Could you check a few things on this model? Use its own coordinates, in mm. A direction names the side the tool comes from. Give positions to 0.01 mm unless a question says otherwise; leave off trailing zeros. Loops run counter-clockwise (first coordinate to the right, second up) from the corner with the lowest first, then second, coordinate; pieces in that order, holes last. Notation, with made-up numbers: (-0.5, 24) - (36.5, 24) arc R34 cw to (36.5, 61) - close; hole circle Ø8 at (-14.5, 68.25). An arc over 180 degrees is marked (long way). Use CSV: the item, a comma, the result in double quotes.
from build123d import *
from OCP.BRepFilletAPI import BRepFilletAPI_MakeChamfer

# Parameters (mm, degrees)
SKIZZE1_R                            = 35
AUFSATZ_LINEAR_AUSTRAGEN1_DEPTH      = 10
SKIZZE1_3_OUTSIDE_W                  = 91.9
SKIZZE1_3_OUTSIDE_H                  = 91.9
SKIZZE1_3_OUTSIDE_R                  = 35
SKIZZE1_3_OUTSIDE_W_2                = 15.1
SKIZZE1_3_OUTSIDE_H_2                = 20.2
SCHNITT_LINEAR_AUSTRAGEN1_DEPTH      = 10
SCHNITT_LINEAR_AUSTRAGEN2_DEPTH      = 1
SCHNITT_LINEAR_AUSTRAGEN2_DEPTH_BACK = 8
SKIZZE2_R                            = 5.1
SKIZZE3_R                            = 32.5
SKIZZE3_R_2                          = 30.5
AUFSATZ_LINEAR_AUSTRAGEN2_DEPTH      = 1
SKIZZE4_R                            = 15.137010129
SKIZZE4_R_2                          = 12.637010129
AUFSATZ_LINEAR_AUSTRAGEN3_DEPTH      = 1
FASE1_SIZE                           = 1
FASE1_SIZE2                          = 5.67128182


with BuildPart() as part:
    # Skizze1 → Aufsatz-Linear austragen1 (new body)
    with BuildSketch(Plane.XY):
        Circle(SKIZZE1_R)
    extrude(amount=AUFSATZ_LINEAR_AUSTRAGEN1_DEPTH)

    # Skizze1_3 outside → Schnitt-Linear austragen1 (cut)
    # profile 1 of 2: a face of its own
    with BuildSketch(Plane.XY):
        Rectangle(SKIZZE1_3_OUTSIDE_W, SKIZZE1_3_OUTSIDE_H)
        Circle(SKIZZE1_3_OUTSIDE_R, mode=Mode.SUBTRACT)
    # profile 2 of 2: a face of its own
    with BuildSketch(Plane.XY):
        with Locations((0.045, 0)):
            Rectangle(SKIZZE1_3_OUTSIDE_W_2, SKIZZE1_3_OUTSIDE_H_2)
    extrude(amount=SCHNITT_LINEAR_AUSTRAGEN1_DEPTH, mode=Mode.SUBTRACT)

    # Skizze2 → Schnitt-Linear austragen2 (cut, two sides: drawn at the far end of the back side and taken through both)
    with BuildSketch(Plane(origin=(0, 0, 0), x_dir=(-1, 0, 0), z_dir=(0, 0, -1)).offset(-SCHNITT_LINEAR_AUSTRAGEN2_DEPTH_BACK)):
        with Locations(Location((0, 25, 0), (0, 0, 180))):
            Circle(SKIZZE2_R)
    extrude(amount=SCHNITT_LINEAR_AUSTRAGEN2_DEPTH + SCHNITT_LINEAR_AUSTRAGEN2_DEPTH_BACK, mode=Mode.SUBTRACT)

    # Skizze3 → Aufsatz-Linear austragen2 (add)
    with BuildSketch(Plane.XY.offset(10)):
        Circle(SKIZZE3_R)
        Circle(SKIZZE3_R_2, mode=Mode.SUBTRACT)
    extrude(amount=AUFSATZ_LINEAR_AUSTRAGEN2_DEPTH)

    # Skizze4 → Aufsatz-Linear austragen3 (add)
    with BuildSketch(Plane.XY.offset(10)):
        Circle(SKIZZE4_R)
        with Locations(Location((0, 0, 0), (0, 0, 53.057558872))):
            Circle(SKIZZE4_R_2, mode=Mode.SUBTRACT)
    extrude(amount=AUFSATZ_LINEAR_AUSTRAGEN3_DEPTH)

    # Fase1: one chamfer whose edges measure the first distance from different faces: ONE call of the kernel's chamfer builder (chamfer() names one face for all edges)
    fase1_edges_1 = [part.edges().sort_by_distance(p)[0] for p in [
        (-7.505, 0, 0),
    ]]
    fase1_side_1 = [part.faces().sort_by_distance(p)[0] for p in [
        (-7.505, 0, 5),
    ]]
    fase1_edges_2 = [part.edges().sort_by_distance(p)[0] for p in [
        (0.045, -10.1, 0),
    ]]
    fase1_side_2 = [part.faces().sort_by_distance(p)[0] for p in [
        (0.045, -10.1, 5),
    ]]
    fase1_edges_3 = [part.edges().sort_by_distance(p)[0] for p in [
        (7.595, 0, 0),
    ]]
    fase1_side_3 = [part.faces().sort_by_distance(p)[0] for p in [
        (7.595, 0, 5),
    ]]
    fase1_edges_4 = [part.edges().sort_by_distance(p)[0] for p in [
        (0.045, 10.1, 0),
    ]]
    fase1_side_4 = [part.faces().sort_by_distance(p)[0] for p in [
        (0.045, 10.1, 5),
    ]]
    fase1 = BRepFilletAPI_MakeChamfer(part.part.solid().wrapped)
    for e in fase1_edges_1:
        fase1.Add(FASE1_SIZE, FASE1_SIZE2, e.wrapped, fase1_side_1[0].wrapped)  # the first distance lies on this face
    for e in fase1_edges_2:
        fase1.Add(FASE1_SIZE, FASE1_SIZE2, e.wrapped, fase1_side_2[0].wrapped)  # the first distance lies on this face
    for e in fase1_edges_3:
        fase1.Add(FASE1_SIZE, FASE1_SIZE2, e.wrapped, fase1_side_3[0].wrapped)  # the first distance lies on this face
    for e in fase1_edges_4:
        fase1.Add(FASE1_SIZE, FASE1_SIZE2, e.wrapped, fase1_side_4[0].wrapped)  # the first distance lies on this face
    add(Compound.cast(fase1.Shape()), mode=Mode.REPLACE)


solid = part.part
1) Suppose I cut it at B-B (y = 0). Please give me the cut outline in (x, z) (3 decimals).
Answer below:
outline,"(-35, 0) - (-13.176, 0) - (-7.505, 1) - (-7.505, 10) - (-12.637, 10) - (-12.637, 11) - (-15.137, 11) - (-15.137, 10) - (-30.5, 10) - (-30.5, 11) - (-32.5, 11) - (-32.5, 10) - (-35, 10) - close; (7.595, 1) - (13.266, 0) - (35, 0) - (35, 10) - (32.5, 10) - (32.5, 11) - (30.5, 11) - (30.5, 10) - (15.137, 10) - (15.137, 11) - (12.637, 11) - (12.637, 10) - (7.595, 10) - close"
2) We'd pull the mould along Y, two halves only. Please class faces 5 (the cylindrical face through (31, 9.76, 10.49)), 6 (the flat face through (-8, 0, 10)), 7 (the flat face through (8, -10, 11)): +Y half, -Y half, draft (parallel to the pull), parting line (faces both ways), or undercut.
Answer below:
face 5,"parting line"
face 6,"undercut"
face 7,"draft"
3) Suppose I cut it at D-D (x = 29.5). Please give me the cut outline in (y, z), plus the area to 3 significant figures.
Answer below:
outline,"(-18.83, 0) - (18.83, 0) - (18.83, 10) - (13.64, 10) - (13.64, 11) - (7.75, 11) - (7.75, 10) - (-7.75, 10) - (-7.75, 11) - (-13.64, 11) - (-13.64, 10) - (-18.83, 10) - close"
area,"388 mm2"
4) I need wall thicknesses on line 1 along Y through (x, z) = (0, 6.25); line 2 along Y through (x, z) = (0, 10.5); line 3 along Y through (x, z) = (-10.5, 10.25). Which ranges of each line are inside material? Lowest first, please.
Answer below:
line 1,"y = -35 to -10.1, 10.1 to 19.9, 30.1 to 35"
line 2,"y = -32.5 to -30.5, -15.14 to -12.64, 12.64 to 15.14, 30.5 to 32.5"
line 3,"y = -30.76 to -28.64, -10.9 to -7.03, 7.03 to 10.9, 28.64 to 30.76"
5) I'm going to push flat-ended pins straight in: P1, Ø8, axis at x = 5, y = 4.5, coming from the +Z side; P2, Ø5, axis at y = 2.5, z = 4.5, coming from the -X side; P3, Ø3, axis at x = -2, y = 24.5, coming from the -Z side; P4, Ø3, axis at y = 23, z = 7, coming from the +X side. Where does each tip first touch, or does it pass through?
Answer below:
P1,"stops at z = 10"
P2,"stops at x = -35"
P3,"stops at z = 8"
P4,"stops at x = 27.62"
6) Which directions (+Z, -Z, +X, -X, +Y, -Y) give clear straight access to the entire face, cutting with the end or side of a thin tool? Please do faces 1 (the flat face through (15, 0, 0)), 2 (the cylindrical face through (-24.204, -18.559, 10.493)), 3 (the flat face through (-7.505, 0, 5)), 4 (the flat face through (0, 25, 8)).
Answer below:
face 1,"-Z, +X, -X, +Y, -Y"
face 2,"+Z"
face 3,"+Z, -Z"
face 4,"-Z"
7) Suppose I cut it at C-C (z = 5.75). Please give me the cut outline in (x, y) (3 decimals).
Answer below:
outline,"circle Ø70 at (0, 0); hole (-7.505, -10.1) - (7.595, -10.1) - (7.595, 10.1) - (-7.505, 10.1) - close; hole circle Ø10.2 at (0, 25)"
